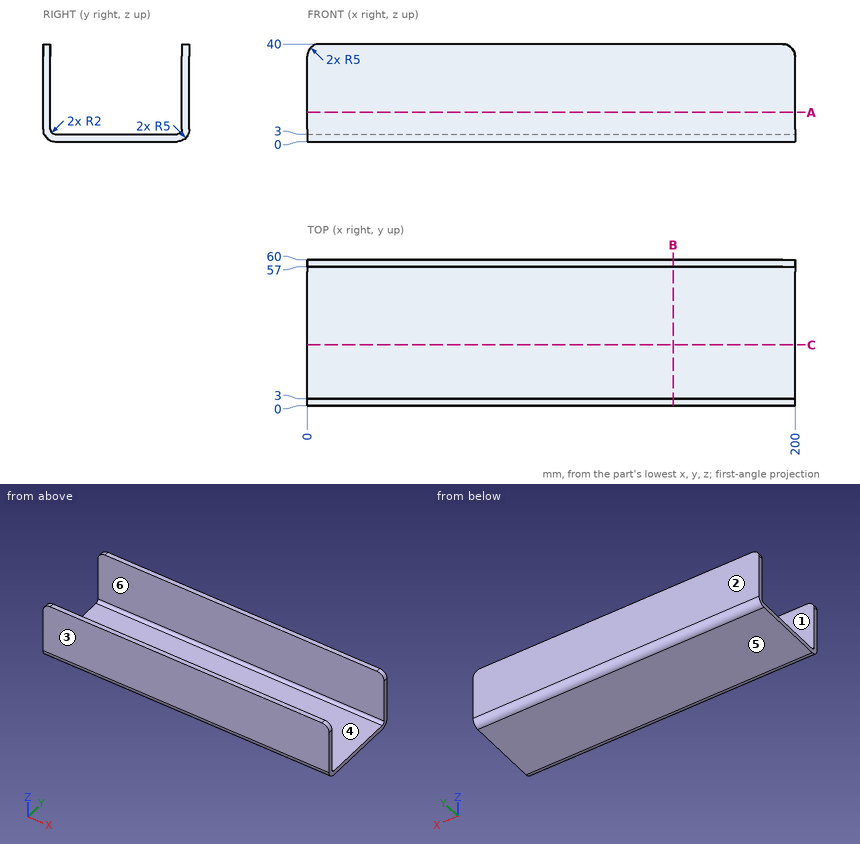
Part print with two shaded views. Sizes in mm from the minimum x, y, z corner. A direction names the side the tool comes from. Round coordinates to 2 decimals unless told otherwise and drop trailing zeros. Order: outer loops, then holes, each group sorted by start corner. A loop starts at its lowest first (then second) coordinate and runs counter-clockwise, first axis right, second up. Notation, with made-up numbers: M 4,-12.75 L 10,-12.75 A9 cw 10,-6.75 Z; hole C 86,16.5 d3. An arc over 180 degrees is marked long. Use CSV: the item, a comma, the result in double quotes. Start each with the question number.
(1) Cut at C-C on y = 25. List the corners of the cut face in (x, z), then the cut area to 3 significant figures.
(2) Cut at B-B on x = 150. List the corners of the cut face in (y, z).
(3) Drill centre lines: probe 1 along Y at (x, z) = (96, 34); probe 2 along Z at (x, y) = (124.5, 15); probe 3 along Y at (x, z) = (127.5, 4). Where is each one in solid material? Low to high.
(4) Flat gauge pin, fed straight in: P1, Ø3, axis at x = 152.5, y = 28, coming from the +Z side. Where does the tip first touch, or does it go through?
(5) Cut at A-A on z = 12. List the corners of the cut face in (x, y), then the cut area to 3 significant figures.
(6) Mould opens along Y. For the marked faces 1, 2, 3 and 4 say: +Y half, -Y half, draft (parallel to the pull), parting line (faces both ways), or undercut.
(7) Tool access for the marked faces 5 and 6: list every direction of +Z, -Z, +X, -X, +Y, -Y with a clear straight run to the whole face (end or side of a thin tool).
Findings:
1,outline,"M 0,0 L 200,0 L 200,3 L 0,3 Z"
1,area,"600 mm^2"
2,outline,"M 0,5 A5 ccw 5,0 L 55,0 A5 ccw 60,5 L 60,40 L 57,40 L 57,5 A2 cw 55,3 L 5,3 A2 cw 3,5 L 3,40 L 0,40 Z"
3,probe 1,"y = 0 to 3, 57 to 60"
3,probe 2,"z = 0 to 3"
3,probe 3,"y = 0.1 to 3.27, 56.73 to 59.9"
4,P1,"stops at z = 3"
5,outline,"M 0,0 L 200,0 L 200,3 L 0,3 Z; M 0,57 L 200,57 L 200,60 L 0,60 Z"
5,area,"1,200 mm^2"
6,face 1,"undercut"
6,face 2,"+Y half"
6,face 3,"-Y half"
6,face 4,"undercut"
7,face 5,"-Z, +X, -X, +Y, -Y"
7,face 6,"+Z, +X, -X"
